Model file for the job. Use its own axes, mm. Face numbers are marked on the shaded views. A direction names the side the tool comes from. Round coordinates to 2 decimals unless told otherwise and drop trailing zeros. Loops run counter-clockwise (first coordinate to the right, second up) from the corner with the lowest first, then second, coordinate; pieces in that order, holes last. Notation, with made-up numbers: M 27,-34.75 L 53,-34.75 A17 cw 53,-13.75 Z; hole C 28,88.5 d6. An arc over 180 degrees is marked long. Use a Markdown table: item, result. Add a question column.
Q1. Cut at D-D (x = -14). Give the cut face in (y, z), plus the area to 3 significant figures.
Q2. Tool access for the marked faces 1, 2, 3 and 4: list every direction of +Z, -Z, +X, -X, +Y, -Y with a clear straight run to the whole face (end or side of a thin tool).
Q3. Cut at A-A (y = 34.5). Give the cut face in (x, z), plus the area to 3 significant figures.
Q4. Cut at C-C (x = 7). Give the cut face in (y, z).
Q5. Mould opens along Z. For the marked faces 5, 6, 7 and 8 say: +Z half, -Z half, draft (parallel to the pull), parting line (faces both ways), or undercut.
Q6. Probe line 1 (Z direction, x = 17.5, y = 24.5); line 2 (X direction, y = 11.5, z = 8); line 3 (Y direction, x = 6, z = -12.5). List the from-to ranges inside material, lowest first. Write a range as from..to.
Q7. Cut at B-B (z = 16.5). Give the cut face in (x, y), plus the area to 3 significant figures.
Q8. Pin check, flat tips, straight feed: pin 1 (8 mm diameter, centred on x = -10, y = 27, fed in from -Z); pin 2 (6 mm diameter, centred on x = 0, z = -16.5, fed in from +Y); pin 3 (3 mm diameter, centred on y = 6, z = 6.5, fed in from -X); pin 4 (6 mm diameter, centred on x = -1.5, z = 10.5, fed in from +Y). Stop position of each tip, or through.
from build123d import *

# Parameters (mm, degrees)
SKETCH1_W           = 5.08
SKETCH1_H           = 8.128
BOSS_EXTRUDE1_DEPTH = 25.4
SKETCH2_W           = 5.08
SKETCH2_H           = 19.05
SKETCH2_W_2         = 7.62
SKETCH2_W_3         = 45.72
SKETCH2_R           = 2.413
BOSS_EXTRUDE2_DEPTH = 0.508
SKETCH2_3_W         = 45.72
SKETCH2_3_H         = 19.05
SKETCH2_3_R         = 2.413
BOSS_EXTRUDE3_DEPTH = 25.4
SKETCH3_W           = 5.588
SKETCH3_H           = 8.128
BOSS_EXTRUDE6_DEPTH = 24.892
FILLET1_R           = 2.54
FILLET2_R           = 2.54
BOSS_EXTRUDE7_DEPTH = 6.35


with BuildPart() as part:
    # Sketch1 → Boss-Extrude1 (new body)
    with BuildSketch(Plane(origin=(0, 0, 0), x_dir=(0, 0, -1), z_dir=(1, 0, 0))):
        Polygon((-33.416737041, 19.05), (-33.416737041, 0), (-15.128737041, 0), (-15.128737041, 10.922), (-20.208737041, 10.922), (-25.796737041, 10.922), (-25.796737041, 19.05), align=None)
        with Locations((-17.668737041, 14.986)):
            Rectangle(SKETCH1_W, SKETCH1_H)
    extrude(amount=-BOSS_EXTRUDE1_DEPTH)

    # Sketch2 → Boss-Extrude2 (add)
    # profile 1 of 4: a face of its own
    with BuildSketch(Plane(origin=(0, 0, 0), x_dir=(0, 0, -1), z_dir=(1, 0, 0))):
        Polygon((-33.416737041, 0), (-15.128737041, 0), (-15.128737041, 19.05), (-20.208737041, 19.05), (-20.208737041, 10.922), (-25.796737041, 10.922), (-25.796737041, 19.05), (-33.416737041, 19.05), align=None)
    # profile 2 of 4: a face of its own
    with BuildSketch(Plane(origin=(0, 0, 0), x_dir=(0, 0, -1), z_dir=(1, 0, 0))):
        with Locations((-17.668737041, 28.575)):
            Rectangle(SKETCH2_W, SKETCH2_H)
    # profile 3 of 4: a face of its own
    with BuildSketch(Plane(origin=(0, 0, 0), x_dir=(0, 0, -1), z_dir=(1, 0, 0))):
        with Locations((-29.606737041, 28.575)):
            Rectangle(SKETCH2_W_2, SKETCH2_H)
    # profile 4 of 4: a face of its own
    with BuildSketch(Plane(origin=(0, 0, 0), x_dir=(0, 0, -1), z_dir=(1, 0, 0))):
        with Locations((7.731262959, 9.525)):
            Rectangle(SKETCH2_W_3, SKETCH2_H)
        with Locations((17.891262959, 14.732)):
            Circle(SKETCH2_R, mode=Mode.SUBTRACT)
    extrude(amount=BOSS_EXTRUDE2_DEPTH)

    # Sketch2<3> → Boss-Extrude3 (add)
    with BuildSketch(Plane(origin=(0, 0, 0), x_dir=(0, 0, -1), z_dir=(1, 0, 0))):
        with Locations((7.731262959, 9.525)):
            Rectangle(SKETCH2_3_W, SKETCH2_3_H)
        with Locations((17.891262959, 14.732)):
            Circle(SKETCH2_3_R, mode=Mode.SUBTRACT)
    extrude(amount=BOSS_EXTRUDE3_DEPTH)

    # Sketch3 → Boss-Extrude6 (add)
    with BuildSketch(Plane(origin=(0.508, 0, 0), x_dir=(0, 0, -1), z_dir=(1, 0, 0))):
        Polygon((-33.416737041, 0), (-15.128737041, 0), (-15.128737041, 19.05), (-15.128737041, 38.1), (-20.208737041, 38.1), (-20.208737041, 10.922), (-25.796737041, 10.922), (-25.796737041, 38.1), (-33.416737041, 38.1), align=None)
        with Locations((-23.002737041, 14.986)):
            Rectangle(SKETCH3_W, SKETCH3_H)
    extrude(amount=BOSS_EXTRUDE6_DEPTH)

    # Fillet1
    # the kernel refuses this fillet: 2.54 mm, written as the material it adds along each edge
    with BuildSketch(Plane(origin=(0, 19.05, 19.446737041), x_dir=(0, 1, 0), z_dir=(0, 0, 1))) as fillet1_piece_1_section:
        with BuildLine():
            CenterArc((FILLET1_R, FILLET1_R), FILLET1_R, 180, 90)
            Line((0, FILLET1_R), (0, 0))
            Line((0, 0), (FILLET1_R, 0))
        make_face()
    fillet1_piece_1 = extrude(amount=13.97, mode=Mode.PRIVATE)
    fillet1_piece_1 = split(fillet1_piece_1, bisect_by=Plane(origin=(-0.57504359, 19.62504359, 20.208737041), z_dir=(0, 0, -1)), keep=Keep.TOP, mode=Mode.PRIVATE)
    add(fillet1_piece_1)
    with BuildSketch(Plane(origin=(0, 19.05, 25.796737041), x_dir=(0, 1, 0), z_dir=(0, 0, 1))) as fillet1_piece_2:
        with BuildLine():
            CenterArc((FILLET1_R, FILLET1_R), FILLET1_R, 180, 90)
            Line((0, FILLET1_R), (0, 0))
            Line((0, 0), (FILLET1_R, 0))
        make_face()
    extrude(amount=7.62)
    with BuildSketch(Plane(origin=(0, 19.05, 15.128737041), x_dir=(0, 1, 0), z_dir=(0, 0, 1))) as fillet1_piece_3:
        with BuildLine():
            CenterArc((FILLET1_R, FILLET1_R), FILLET1_R, 180, 90)
            Line((0, FILLET1_R), (0, 0))
            Line((0, 0), (FILLET1_R, 0))
        make_face()
    extrude(amount=5.08)
    with BuildSketch(Plane(origin=(0, 19.05, 15.128737041), x_dir=(0, 1, 0), z_dir=(0, 0, 1))) as fillet1_piece_4_section:
        with BuildLine():
            CenterArc((FILLET1_R, FILLET1_R), FILLET1_R, 180, 90)
            Line((0, FILLET1_R), (0, 0))
            Line((0, 0), (FILLET1_R, 0))
        make_face()
    fillet1_piece_4 = extrude(amount=11.43, mode=Mode.PRIVATE)
    fillet1_piece_4 = split(fillet1_piece_4, bisect_by=Plane(origin=(-0.57504359, 19.62504359, 25.796737041), z_dir=(0, 0, 1)), keep=Keep.TOP, mode=Mode.PRIVATE)
    add(fillet1_piece_4)

    # Fillet2
    fillet2_edges = [part.edges().sort_by_distance(p)[0] for p in [
        (12.7, 19.05, -30.591262959),
    ]]
    fillet(fillet2_edges, radius=FILLET2_R)

    # Sketch4 → Boss-Extrude7 (add)
    with BuildSketch(Plane.XZ):
        Polygon((0.508, 28.082737041), (0.508, 24.272737041), (0.508, 20.462737041), (25.4, 20.462737041), (25.4, 24.272737041), (25.4, 28.082737041), align=None)
        Polygon((25.4, -13.827262959), (25.4, -10.017262959), (0.508, -10.017262959), (0.508, -17.637262959), (25.4, -17.637262959), align=None)
    extrude(amount=BOSS_EXTRUDE7_DEPTH)


solid = part.part
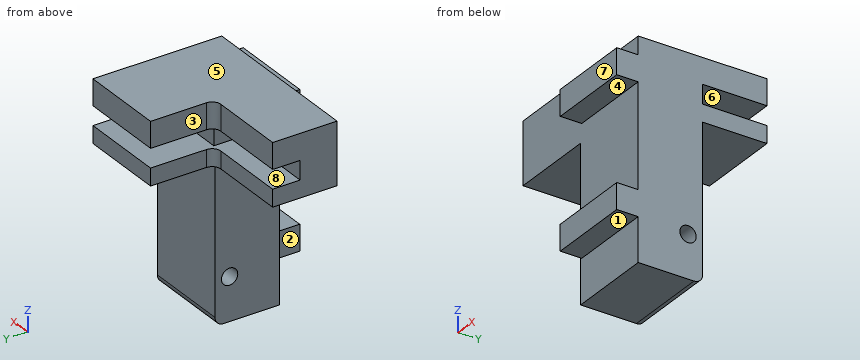
Checked values:
| question | item | result |
|---|---|---|
| 1 | outline | M 0,15.13 L 19.05,15.13 L 19.05,20.21 L 10.92,20.21 L 10.92,25.8 L 19.05,25.8 L 19.05,33.42 L 0,33.42 Z |
| 1 | area | 303 mm^2 |
| 2 | face 1 | -Z, +X, -X, -Y |
| 2 | face 2 | +Z, -Z, -X, -Y |
| 2 | face 3 | +Z, -Z, -X, +Y |
| 2 | face 4 | +X, -X, -Y |
| 3 | outline | M 0,15.13 L 25.4,15.13 L 25.4,20.21 L 0,20.21 Z; M 0,25.8 L 25.4,25.8 L 25.4,33.42 L 0,33.42 Z |
| 3 | area | 323 mm^2 |
| 4 | outline | M -6.35,-17.64 L 0,-17.64 L 0,-30.59 L 16.51,-30.59 A2.54 ccw 19.05,-28.05 L 19.05,15.13 L 38.1,15.13 L 38.1,20.21 L 19.05,20.21 L 19.05,25.8 L 38.1,25.8 L 38.1,33.42 L 0,33.42 L 0,28.08 L -6.35,28.08 L -6.35,20.46 L 0,20.46 L 0,-10.02 L -6.35,-10.02 Z; hole C 14.73,-17.89 d4.83 |
| 5 | face 5 | +Z half |
| 5 | face 6 | undercut |
| 5 | face 7 | draft |
| 5 | face 8 | undercut |
| 6 | line 1 | z = 15.13..20.21, 25.8..33.42 |
| 6 | line 2 | x = 0..25.4 |
| 6 | line 3 | y = -6.35..19.05 |
| 7 | outline | M -25.4,0 L 25.4,0 L 25.4,38.1 L 0,38.1 L 0,21.59 A2.54 cw -2.54,19.05 L -25.4,19.05 Z |
| 7 | area | 1,450 mm^2 |
| 8 | pin 1 | passes through |
| 8 | pin 2 | stops at y = 19.05 |
| 8 | pin 3 | stops at x = 0 |
| 8 | pin 4 | stops at y = 19.05 |
